Source: three-view drawing plus pictorial views. Frame: mm from the lowest corner of the part. A direction names the side the tool comes from. Coordinates: 2 decimals unless noted, no trailing zeros. Write each loop counter-clockwise with the first axis right and the second up, starting at its lowest first coordinate (ties: lowest second). Pieces come first, ordered by that corner, then holes. Notation, with made-up numbers: (16, -19) - (72, -19) arc R14 ccw to (72, 0) - close; hole circle Ø4 at (65.25, 0.5). An arc over 180 degrees is marked (long way). Put each result on its own line as item: value. Start each with the question number.
1. Cut plane A-A, the plane y = 23. Return loops of the section in (x, z).
2. Pin query (flat end, axial travel): pin 1 (12 mm diameter, centred on y = 21, z = 42.5, fed in from +X); pin 2 (5 mm diameter, centred on y = 24.5, z = 97, fed in from -X); pin 3 (5 mm diameter, centred on x = 52, z = 24, fed in from -Y); pin 4 (3 mm diameter, centred on x = 57.5, y = 24.5, fed in from -Z). Return the tip coordinate at first contact, or that it passes through.
3. Cut plane C-C, the plane x = 58. Return loops of the section in (y, z), and give its area (3 significant figures).
4. Line query: line 1 (Z direction, x = 63.5, y = 8.5); line 2 (X direction, y = 27.25, z = 58); line 3 (X direction, y = 27.75, z = 9.5). Output: solid intervals per line, ascending.
5. Cut plane B-B, the plane z = 58. Return loops of the section in (x, y).
6. Access query for the marked faces 1 and 2. Directions: +Z, -Z, +X, -X, +Y, -Y. A direction counts if a zero-diameter tool reaches every point of the face in a straight line with its end or side. Return the directions, or none.
7. Cut plane D-D, the plane y = 6.75. Return loops of the section in (x, z).
8. Pull-direction query (Z, two-part tool) for the marked faces 3, 4 and 5; classes: released by +Z, released by -Z, zero draft, split by the parting line, or undercut.
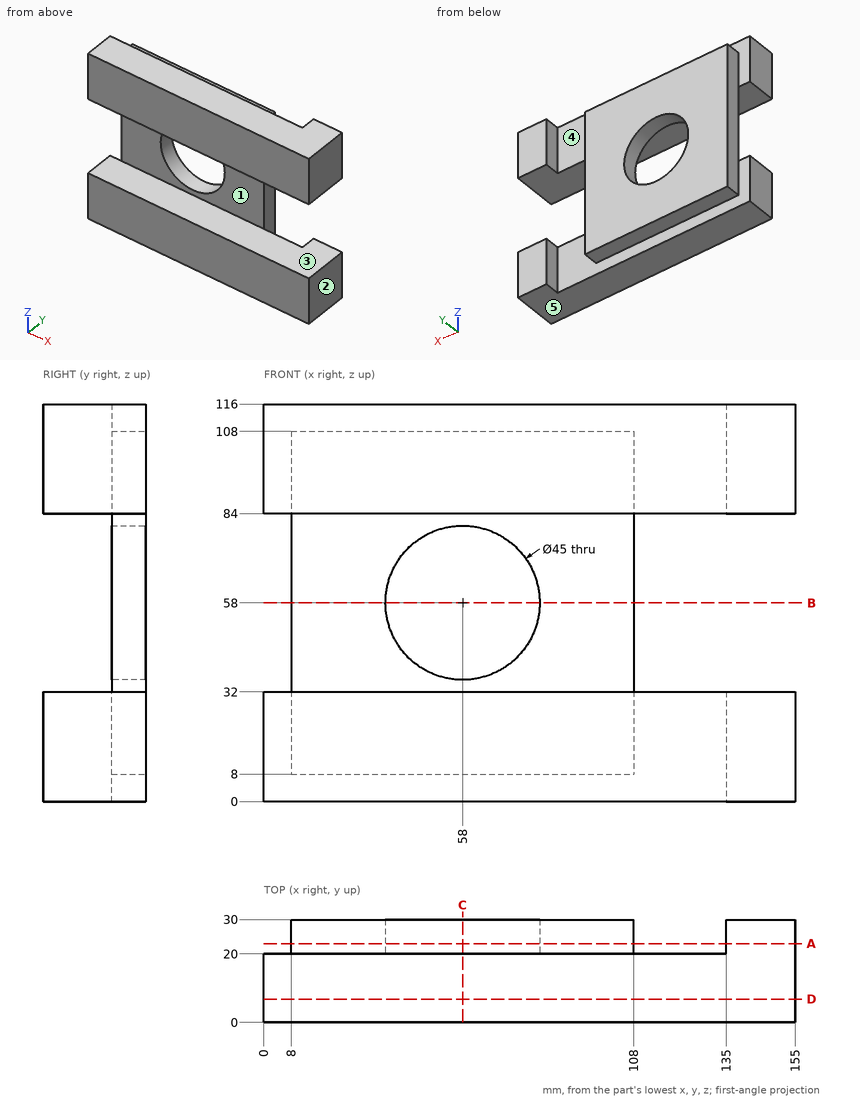
Report:
1. outline: (8, 8) - (108, 8) - (108, 108) - (8, 108) - close; (135, 0) - (155, 0) - (155, 32) - (135, 32) - close; (135, 84) - (155, 84) - (155, 116) - (135, 116) - close; hole circle Ø45 at (58, 58)
2. pin 1: stops at x = 108
2. pin 2: stops at x = 8
2. pin 3: stops at y = 0
2. pin 4: stops at z = 8
3. outline: (0, 0) - (20, 0) - (20, 8) - (30, 8) - (30, 35.5) - (20, 35.5) - (20, 32) - (0, 32) - close; (0, 84) - (20, 84) - (20, 80.5) - (30, 80.5) - (30, 108) - (20, 108) - (20, 116) - (0, 116) - close
3. area: 1,830 mm^2
4. line 1: z = 0 to 32, 84 to 116
4. line 2: x = 8 to 35.5, 80.5 to 108
4. line 3: x = 8 to 108, 135 to 155
5. outline: (8, 20) - (35.5, 20) - (35.5, 30) - (8, 30) - close; (80.5, 20) - (108, 20) - (108, 30) - (80.5, 30) - close
6. face 1: +X, -X, -Y
6. face 2: +Z, -Z, +X, +Y, -Y
7. outline: (0, 0) - (155, 0) - (155, 32) - (0, 32) - close; (0, 84) - (155, 84) - (155, 116) - (0, 116) - close
8. face 3: undercut
8. face 4: zero draft
8. face 5: released by -Z
